Geometry check sheet. Reference: the model listing, model coordinates, mm. Face numbers are marked on the shaded views. A direction names the side the tool comes from. Give positions to 0.01 mm unless a question says otherwise; leave off trailing zeros. Write each loop counter-clockwise with the first axis right and the second up, starting at its lowest first coordinate (ties: lowest second). Pieces come first, ordered by that corner, then holes. Notation, with made-up numbers: M -23,-30 L 29,-30 A19 ccw 29,-2 Z; hole C 58,-13 d4. An arc over 180 degrees is marked long. One line per item, written item: value. Start each with the question number.
1. Cross-section at A-A on z = -11. Record the cut outline in (x, y), then the cut area to 3 significant figures.
2. Release check for a two-part mould opening along Y. For the marked faces 4, 5 and 6 record: pulls with the +Y half, pulls with the -Y half, needs draft (parallel to the pull), parting line crosses it, or undercut.
3. Tool access check on the marked faces 1, 2 and 3. Record the directions out of +Z, -Z, +X, -X, +Y, -Y that give a thin tool (end or side, any length) a straight path to the whole face; none if there is none.
4. Cross-section at B-B on y = 0. Count the separate pieces of the cut face and the enclosed holes in it, then the cut area to 3 significant figures.
5. Gauge pin test, flat ends, axial feed: pin 1 (4 mm diameter, centred on x = -10, z = -11, fed in from +Y); pin 2 (1.5 mm diameter, centred on x = -1, z = -6.5, fed in from -Y); pin 3 (1 mm diameter, centred on y = 6, z = -6.5, fed in from -X) (3 decimals). Record the tip position at first contact, or that the pin passes through.
6. Scan lines: line 1 (Y direction, x = 0.25, z = -7); line 2 (X direction, y = -2, z = -9); line 3 (X direction, y = 5.5, z = -0.75). Record each from-to range of solid material in increasing order.
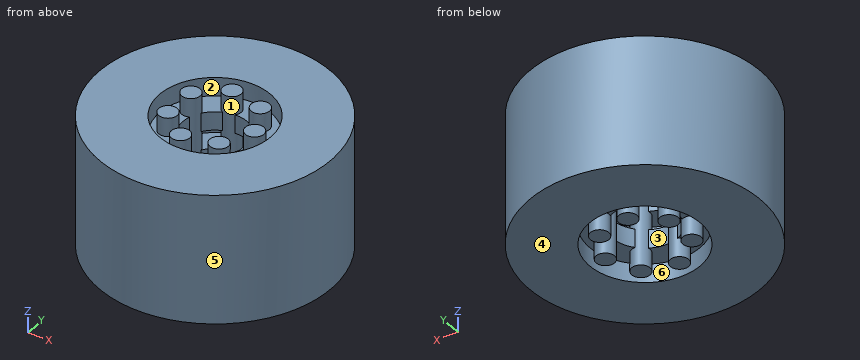
Autodesk Inventor part; units mm, degrees
ref_plane "YZ Plane" through (0, 0, 0) normal (1, 0, 0) x (0, 1, 0)
ref_plane "XZ Plane" through (0, 0, 0) normal (0, 1, 0) x (-1, 0, 0)
ref_plane "XY Plane" through (0, 0, 0) normal (0, 0, 1) x (1, 0, 0)
sketch "Sketch1" plane through (0, 0, 0) normal (1, 0, 0) x (0, 1, 0)
  line L0 (3.5, -4) -> (3.5, -2)
  line L1 (6, -2) -> (6, 0)
  line L2 (6, -6) -> (6, -4)
  line L3 (3.5, -8) -> (3.5, -6)
  line L4 (6, -10) -> (6, -8)
  line L5 (3.4951, -12) -> (3.4951, -10)
  line L6 (6, -14) -> (6, -12)
  line L7 (0, 0) -> (0, -14)
  line L8 (6, 0) -> (12.5, 0)
  line L9 (12.5, 0) -> (12.5, -14)
  line L10 (12.5, -14) -> (6, -14)
  line L11 (6, -12) -> (3.4951, -12)
  line L12 (3.4951, -10) -> (6, -10)
  line L13 (6, -8) -> (3.5, -8)
  line L14 (3.5, -6) -> (6, -6)
  line L15 (6, -4) -> (3.5, -4)
  line L16 (3.5, -2) -> (6, -2)
  point P0 (9.25, 0)
  dimension "d1" = 12.5
revolve "Revolution1" add sketch "Sketch1" angle 360 about axis through (0, 0, 0) along (0, 0, -1)
sketch "Sketch2" plane through (0, 0, 0) normal (0, 0, 1) x (1, 0, 0)
  circle A0 centre (-0.9457, -4.1434) radius 1
  circle A1 centre (-3.8291, 1.844) radius 1
  circle A2 centre (2.6498, 3.3228) radius 1
  circle A3 centre (4.25, 0) radius 1
  circle A4 centre (-0.9457, 4.1434) radius 1
  circle A5 centre (-3.8291, -1.844) radius 1
  circle A6 centre (2.6498, -3.3228) radius 1
  circle A7 centre (0, 0) radius 6
  point P0 (0, 0)
extrude "Extrusion1" add sketch "Sketch2" against normal up to surface (14 mm away) contours A0 | A1 | A2 | A3 | A4 | A5 | A6
properties part number "opona" material "Rubber, Silicone"
Report:
1. outline: C 0,0 d25; hole M -3.36,-0.96 A1 cw -2.85,-2.03 A3.5 ccw -1.34,-3.23 A1 cw -0.19,-3.49 A3.5 ccw 1.68,-3.06 A1 cw 2.61,-2.32 A3.5 ccw 3.44,-0.59 A1 cw 3.44,0.59 A3.5 ccw 2.61,2.32 A1 cw 1.68,3.06 A3.5 ccw -0.19,3.49 A1 cw -1.34,3.23 A3.5 ccw -2.85,2.03 A1 cw -3.36,0.96 A3.5 ccw Z
1. area: 454 mm^2
2. face 4: needs draft
2. face 5: parting line crosses it
2. face 6: undercut
3. face 1: none
3. face 2: +Z
3. face 3: +Z, -Z
4. separate pieces: 2
4. enclosed holes: 2
4. area: 230 mm^2
5. pin 1: stops at y = 9.6
5. pin 2: stops at y = -12.5
5. pin 3: stops at x = -11.225
6. line 1: y = -12.5 to -3.49, 3.49 to 12.5
6. line 2: x = -12.34 to -5.66, -4.82 to -2.84, 5.66 to 12.34
6. line 3: x = -11.22 to -2.4, 2.4 to 11.22
